Here's how the part is built. I have some questions about the finished solid (model axes, mm). Face numbers are marked on the shaded views. A direction names the side the tool comes from. Coordinates: 2 decimals unless noted, no trailing zeros. Write each loop counter-clockwise with the first axis right and the second up, starting at its lowest first coordinate (ties: lowest second). Pieces come first, ordered by that corner, then holes. Notation, with made-up numbers: (32, 40.25) -> (41, 40.25) arc R17 cw to (41, 71.25) -> close; hole circle Ø8 at (60, -10). An arc over 180 degrees is marked (long way). Use a Markdown table: item, result. Add a question column.
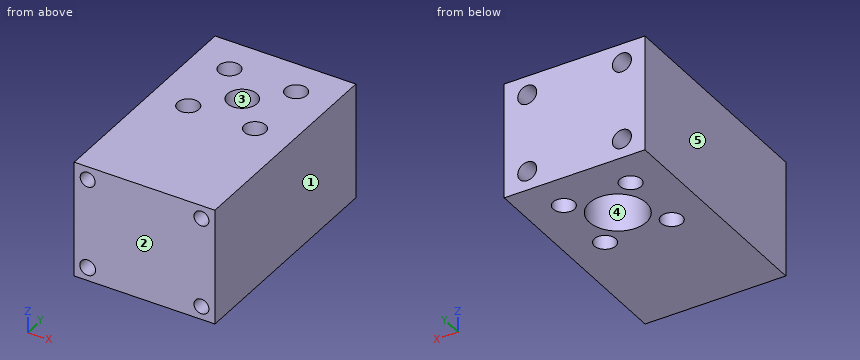
```python
from build123d import *

# Parameters (mm, degrees)
SKETCH1_W           = 47
SKETCH1_H           = 38.8
SKETCH1_R           = 2.5
SKETCH1_R_2         = 2.627
BOSS_EXTRUDE1_DEPTH = 76.2
SKETCH2_R           = 3.571875
SKETCH2_R_2         = 4.92125
CUT_EXTRUDE1_DEPTH  = 39.8
SKETCH1_8_R         = 2.627
SKETCH1_8_R_2       = 2.5
CUT_EXTRUDE2_DEPTH  = 38.1
SKETCH4_R           = 9.525
CUT_EXTRUDE4_DEPTH  = 21.0185
SKETCH5_R           = 3.175
CUT_EXTRUDE5_DEPTH  = 6.35


with BuildPart() as part:
    # Sketch1 → Boss-Extrude1 (new body)
    with BuildSketch(Plane(origin=(0, 0, 0), x_dir=(1, 0, 0), z_dir=(0, 1, 0))):
        with Locations((23.5, 19.4)):
            Rectangle(SKETCH1_W, SKETCH1_H)
        with Locations((4.5, 4.4)):
            Circle(SKETCH1_R, mode=Mode.SUBTRACT)
        with Locations((42.5, 4.4)):
            Circle(SKETCH1_R, mode=Mode.SUBTRACT)
        with Locations((4.5, 34.4)):
            Circle(SKETCH1_R_2, mode=Mode.SUBTRACT)
        with Locations((42.5, 34.4)):
            Circle(SKETCH1_R, mode=Mode.SUBTRACT)
        with Locations((42.5, 4.4)):
            Circle(SKETCH1_R)
        with Locations((4.5, 4.4)):
            Circle(SKETCH1_R)
        with Locations((4.5, 34.4)):
            Circle(SKETCH1_R_2)
        with Locations((42.5, 34.4)):
            Circle(SKETCH1_R)
    extrude(amount=BOSS_EXTRUDE1_DEPTH)

    # Sketch2 → Cut-Extrude1 (cut, through all)
    with BuildSketch(Plane.XY):
        with Locations((12.36448241, 63.94291018)):
            Circle(SKETCH2_R)
        with Locations((34.63551759, 63.94291018)):
            Circle(SKETCH2_R)
        with Locations((34.63551759, 41.671875)):
            Circle(SKETCH2_R)
        with Locations((23.5, 52.80739259)):
            Circle(SKETCH2_R_2)
        with Locations((12.36448241, 41.671875)):
            Circle(SKETCH2_R)
    extrude(amount=-CUT_EXTRUDE1_DEPTH, mode=Mode.SUBTRACT)

    # Sketch1_8 → Cut-Extrude2 (cut)
    with BuildSketch(Plane(origin=(0, 0, 0), x_dir=(1, 0, 0), z_dir=(0, 1, 0))):
        with Locations((4.5, 34.4)):
            Circle(SKETCH1_8_R)
        with Locations((4.5, 4.4)):
            Circle(SKETCH1_8_R_2)
        with Locations((42.5, 4.4)):
            Circle(SKETCH1_8_R_2)
        with Locations((42.5, 34.4)):
            Circle(SKETCH1_8_R_2)
    extrude(amount=CUT_EXTRUDE2_DEPTH, mode=Mode.SUBTRACT)

    # Sketch4 → Cut-Extrude4 (cut)
    with BuildSketch(Plane(origin=(0, 0, -38.8), x_dir=(-1, 0, 0), z_dir=(0, 0, -1))):
        with Locations((-23.5, 52.80739259)):
            Circle(SKETCH4_R)
    extrude(amount=-CUT_EXTRUDE4_DEPTH, mode=Mode.SUBTRACT)

    # Sketch5 → Cut-Extrude5 (cut)
    with BuildSketch(Plane(origin=(0, 76.2, 0), x_dir=(1, 0, 0), z_dir=(0, 1, 0))):
        with Locations((7.692010309, 32.45)):
            Circle(SKETCH5_R)
        with Locations((39.307989691, 32.45)):
            Circle(SKETCH5_R)
        with Locations((39.307989691, 6.35)):
            Circle(SKETCH5_R)
        with Locations((7.692010309, 6.35)):
            Circle(SKETCH5_R)
    extrude(amount=-CUT_EXTRUDE5_DEPTH, mode=Mode.SUBTRACT)


solid = part.part
```
Q1. Suppose I cut it at A-A, the plane y = 34. Write out the boundary of the cut face in (x, z), and give its area (3 significant figures).
Q2. Suppose I cut it at C-C, the plane x = 6. Write out the boundary of the cut face in (y, z), and give its area (3 significant figures).
Q3. Suppose I cut it at B-B, the plane z = -27. Write out the boundary of the cut face in (x, y) (3 decimals), and give its area (3 significant figures).
Q4. Which directions (+Z, -Z, +X, -X, +Y, -Y) give clear straight access to the entire face, cutting with the end or side of a thin tool? Please do the marked faces 4 and 5.
Q5. Please list where these lines run through material, in increasing order: line 1 (X direction, y = 41.5, z = -36); line 2 (Z direction, x = 42.5, y = 21); line 3 (X direction, y = 12, z = -4.4).
Q6. Suppose I cut it at D-D, the plane z = -34.4. Write out the boundary of the cut face in (x, y) (3 decimals), and give its area (3 significant figures).
Q7. Will these pins go through, and if not, where does the flat tip stop? pin 1 (2.5 mm diameter, centred on x = 43, z = -4, fed in from -Y); pin 2 (1.9 mm diameter, centred on x = 7, z = -33, fed in from +Y); pin 3 (13 mm diameter, centred on x = 23.5, y = 52.81, fed in from -Z).
Q8. Thinking about a two-plate mould opening in Y: for the marked faces 1, 2 and 3, which applies, released by +Y, released by -Y, zero draft, split by the parting line, or undercut?
Answer key:
| question | item | result |
|---|---|---|
| 1 | outline | (0, -38.8) -> (47, -38.8) -> (47, 0) -> (0, 0) -> close; hole circle Ø5.25 at (4.5, -34.4); hole circle Ø5 at (4.5, -4.4); hole circle Ø5 at (42.5, -34.4); hole circle Ø5 at (42.5, -4.4) |
| 1 | area | 1,740 mm^2 |
| 2 | outline | (0, -38.8) -> (76.2, -38.8) -> (76.2, -35.14) -> (69.85, -35.14) -> (69.85, -29.76) -> (76.2, -29.76) -> (76.2, -9.04) -> (69.85, -9.04) -> (69.85, -3.66) -> (76.2, -3.66) -> (76.2, 0) -> (0, 0) -> (0, -2.4) -> (38.1, -2.4) -> (38.1, -6.4) -> (0, -6.4) -> (0, -32.24) -> (38.1, -32.24) -> (38.1, -36.56) -> (0, -36.56) -> close |
| 2 | area | 2,570 mm^2 |
| 3 | outline | (0, 0) -> (47, 0) -> (47, 76.2) -> (0, 76.2) -> close; hole circle Ø7.144 at (12.364, 41.672); hole circle Ø7.144 at (12.364, 63.943); hole circle Ø19.05 at (23.5, 52.807); hole circle Ø7.144 at (34.636, 41.672); hole circle Ø7.144 at (34.636, 63.943) |
| 3 | area | 3,140 mm^2 |
| 4 | face 4 | -Z |
| 4 | face 5 | +Z, -Z, -X, +Y, -Y |
| 5 | line 1 | x = 0 to 8.8, 15.93 to 31.07, 38.2 to 47 |
| 5 | line 2 | z = -38.8 to -36.9, -31.9 to -6.9, -1.9 to 0 |
| 5 | line 3 | x = 0 to 2, 7 to 40, 45 to 47 |
| 6 | outline | (0, 0) -> (1.873, 0) -> (1.873, 38.1) -> (7.127, 38.1) -> (7.127, 0) -> (40, 0) -> (40, 38.1) -> (45, 38.1) -> (45, 0) -> (47, 0) -> (47, 76.2) -> (41.814, 76.2) -> (41.814, 69.85) -> (36.802, 69.85) -> (36.802, 76.2) -> (10.198, 76.2) -> (10.198, 69.85) -> (5.186, 69.85) -> (5.186, 76.2) -> (0, 76.2) -> close; hole circle Ø7.144 at (12.364, 41.672); hole circle Ø7.144 at (12.364, 63.943); hole circle Ø19.05 at (23.5, 52.807); hole circle Ø7.144 at (34.636, 41.672); hole circle Ø7.144 at (34.636, 63.943) |
| 6 | area | 2,680 mm^2 |
| 7 | pin 1 | stops at y = 38.1 |
| 7 | pin 2 | stops at y = 69.85 |
| 7 | pin 3 | stops at z = -17.78 |
| 8 | face 1 | zero draft |
| 8 | face 2 | released by -Y |
| 8 | face 3 | undercut |
